```python
from build123d import *

# Parameters (mm, degrees)
SKETCH_1_R               = 28.5
EXTRUDE_1_DEPTH          = 46
SKETCH_2_R               = 17.5
EXTRUDE_2_DEPTH          = 1
SKETCH_4_R               = 1.5
CUT_EXTRUDE_1_DEPTH      = 4
PATTERN_CIRCULAR_1_COUNT = 4
SKETCH_5_R               = 2
CUT_EXTRUDE_2_DEPTH      = 4
PATTERN_CIRCULAR_2_COUNT = 3
SKETCH_6_R               = 1.5
CUT_EXTRUDE_3_DEPTH      = 5
PATTERN_CIRCULAR_3_COUNT = 6
SKETCH_8_R               = 1.5
CUT_EXTRUDE_4_DEPTH      = 5
PATTERN_CIRCULAR_4_COUNT = 6


with BuildPart() as part:
    # 草图1 → 凸台-拉伸1 (new body)
    with BuildSketch(Plane(origin=(0, 0, 0), x_dir=(1, 0, 0), z_dir=(0, 1, 0))):
        with Locations(Location((0, 0, 0), (0, 0, 270))):
            Circle(SKETCH_1_R)
    extrude(amount=EXTRUDE_1_DEPTH)

    # 草图2 → 凸台-拉伸2 (add)
    with BuildSketch(Plane(origin=(0, 46, 0), x_dir=(1, 0, 0), z_dir=(0, 1, 0))):
        with Locations(Location((0, 0, 0), (0, 0, 270))):
            Circle(SKETCH_2_R)
    extrude(amount=EXTRUDE_2_DEPTH)

    # 草图4 → 切除-拉伸1 (cut)
    with BuildSketch(Plane.XZ):
        with Locations(Location((13.435028843, 13.435028843, 0), (0, 0, 270))):
            Circle(SKETCH_4_R)
    cut_extrude_1 = extrude(amount=-CUT_EXTRUDE_1_DEPTH, mode=Mode.SUBTRACT)

    # 阵列(圆周)1: 切除-拉伸1 ×4 about axis
    pattern_circular_1_axis = Axis((0, 0, 0), (0, 1, 0))
    for i in range(1, PATTERN_CIRCULAR_1_COUNT):
        add(cut_extrude_1.rotate(pattern_circular_1_axis, i * 360 / PATTERN_CIRCULAR_1_COUNT), mode=Mode.SUBTRACT)

    # 草图5 → 切除-拉伸2 (cut)
    with BuildSketch(Plane(origin=(0, 47, 0), x_dir=(1, 0, 0), z_dir=(0, 1, 0))):
        with Locations(Location((10.522208656, 6.075, 0), (0, 0, 270))):
            Circle(SKETCH_5_R)
    cut_extrude_2 = extrude(amount=-CUT_EXTRUDE_2_DEPTH, mode=Mode.SUBTRACT)

    # 阵列(圆周)2: 切除-拉伸2 ×3 about axis
    pattern_circular_2_axis = Axis((-0.139251727, 0, 0.080397022), (0, 1, 0))
    for i in range(1, PATTERN_CIRCULAR_2_COUNT):
        add(cut_extrude_2.rotate(pattern_circular_2_axis, i * 360 / PATTERN_CIRCULAR_2_COUNT), mode=Mode.SUBTRACT)

    # 草图6 → 切除-拉伸3 (cut)
    with BuildSketch(Plane(origin=(0, 47, 0), x_dir=(1, 0, 0), z_dir=(0, 1, 0))):
        with Locations(Location((13.5, 0, 0), (0, 0, 270))):
            Circle(SKETCH_6_R)
    cut_extrude_3 = extrude(amount=-CUT_EXTRUDE_3_DEPTH, mode=Mode.SUBTRACT)

    # 阵列(圆周)3: 切除-拉伸3 ×6 about axis
    pattern_circular_3_axis = Axis((0, 0, 0), (0, 1, 0))
    for i in range(1, PATTERN_CIRCULAR_3_COUNT):
        add(cut_extrude_3.rotate(pattern_circular_3_axis, i * 360 / PATTERN_CIRCULAR_3_COUNT), mode=Mode.SUBTRACT)

    # 草图8 → 切除-拉伸4 (cut)
    with BuildSketch(Plane(origin=(0, 46, 0), x_dir=(1, 0, 0), z_dir=(0, 1, 0))):
        with Locations(Location((0, 25, 0), (0, 0, 270))):
            Circle(SKETCH_8_R)
    cut_extrude_4 = extrude(amount=-CUT_EXTRUDE_4_DEPTH, mode=Mode.SUBTRACT)

    # 阵列(圆周)4: 切除-拉伸4 ×6 about axis
    pattern_circular_4_axis = Axis((0, 0, 0), (0, 1, 0))
    for i in range(1, PATTERN_CIRCULAR_4_COUNT):
        add(cut_extrude_4.rotate(pattern_circular_4_axis, i * 360 / PATTERN_CIRCULAR_4_COUNT), mode=Mode.SUBTRACT)


solid = part.part
```
Geometry check sheet. Reference: the model listing, model coordinates, mm. A direction names the side the tool comes from. Round coordinates to 2 decimals unless told otherwise and drop trailing zeros. Loops run counter-clockwise (first coordinate to the right, second up) from the corner with the lowest first, then second, coordinate; pieces in that order, holes last. Notation, with made-up numbers: (41.25, 71.5) -> (98.25, 71.5) arc R30 cw to (98.25, 109.5) -> close; hole circle Ø1 at (2, -22.75). An arc over 180 degrees is marked (long way). Use a Markdown table: item, result.
(1) Sectioned sample at A-A (z = 0). Enter the section's corners in (x, y).
Calculated:
| item | result |
|---|---|
| outline | (-28.5, 0) -> (28.5, 0) -> (28.5, 46) -> (17.5, 46) -> (17.5, 47) -> (15, 47) -> (15, 42) -> (12, 42) -> (12, 47) -> (-12, 47) -> (-12, 42) -> (-15, 42) -> (-15, 47) -> (-17.5, 47) -> (-17.5, 46) -> (-28.5, 46) -> close |
(2) Set-up check for faces 1 (the flat face through (-11, 43, -6)), 2 (the cylindrical face through (-13.886, 1.972, -12.004)): record each of +Z, -Z, +X, -X, +Y, -Y from which the full face is reachable in a straight line by a thin tool's end or side.
Calculated:
| item | result |
|---|---|
| face 1 | +Y |
| face 2 | -Y |
(3) Mould release check, pull along Z, two halves, no side actions. Record for faces 3 (the cylindrical face through (-10.648, 46.493, -13.887)), 4 (the flat face through (13, 4, -13)), 5 (the flat face through (0, 0, 0)), 6 (the flat face through (22, 41, 13)): released by +Z, released by -Z, zero draft, split by the parting line, or undercut.
Calculated:
| item | result |
|---|---|
| face 3 | split by the parting line |
| face 4 | undercut |
| face 5 | zero draft |
| face 6 | undercut |
(4) Scan lines: probe 1 along X at (y, z) = (43.1, 0); probe 2 along Y at (x, z) = (-22, -11.5); probe 3 along X at (y, z) = (42.2, 12.5). Record each from-to range of solid material in increasing order.
Calculated:
| item | result |
|---|---|
| probe 1 | -28.5 to -15, -12 to 12, 15 to 28.5 |
| probe 2 | 0 to 41 |
| probe 3 | -25.61 to -23.15, -20.15 to -8.01, -5.49 to 5.49, 8.01 to 20.15, 23.15 to 25.61 |
(5) Go/stop test with flat-tipped pins: P1, Ø3.5, axis at x = 21.5, z = 12.5, coming from the +Y side; P2, Ø8, axis at y = 41.5, z = -3.5, coming from the -X side; P3, Ø10, axis at x = -12, y = 19, coming from the -Z side. Record where each tip stops, or that it passes through.
Calculated:
| item | result |
|---|---|
| P1 | y = 46 |
| P2 | x = -28.5 |
| P3 | z = -27.63 |
(6) Sectioned sample at B-B (y = 3). Enter the section's corners in (x, z), then the cut area to 3 significant figures.
Calculated:
| item | result |
|---|---|
| outline | circle Ø57 at (0, 0); hole circle Ø3 at (-13.44, -13.44); hole circle Ø3 at (-13.44, 13.44); hole circle Ø3 at (13.44, -13.44); hole circle Ø3 at (13.44, 13.44) |
| area | 2,520 mm² |
(7) Sectioned sample at D-D (y = 30). Enter the section's corners in (x, z), then the cut area to 3 significant figures.
Calculated:
| item | result |
|---|---|
| outline | circle Ø57 at (0, 0) |
| area | 2,550 mm² |
(8) Sectioned sample at C-C (x = 6.75). Enter the section's corners in (y, z), then the cut area to 3 significant figures.
Calculated:
| item | result |
|---|---|
| outline | (0, -27.69) -> (46, -27.69) -> (46, -16.15) -> (47, -16.15) -> (47, -13.19) -> (42, -13.19) -> (42, -10.19) -> (47, -10.19) -> (47, 10.19) -> (42, 10.19) -> (42, 13.19) -> (47, 13.19) -> (47, 16.15) -> (46, 16.15) -> (46, 27.69) -> (0, 27.69) -> close |
| area | 2,550 mm² |
